from build123d import *

# Parameters (mm, degrees)
F0_W     = 40
F0_H     = 20
F1_DEPTH = 20
F3_DEPTH = 40.001


with BuildPart() as f1:
    # F0 (on Top) → F1 (new body)
    with BuildSketch(Plane.XY):
        with Locations((-41.790509, -39.392859)):
            Rectangle(F0_W, F0_H)
    extrude(amount=F1_DEPTH)

    # F2 (on face) → F3 (cut, through all)
    with BuildSketch(Plane.YZ.offset(-21.790509)):
        Polygon((-39.392859, 10), (-39.392859, 20), (-49.392859, 20), (-49.392859, 0), align=None)
    extrude(amount=-F3_DEPTH, mode=Mode.SUBTRACT)


solid = f1.part
The model under review builds one solid part; all positions refer to its coordinate system, in mm. A direction names the side the tool comes from. Coordinates: 2 decimals unless noted, no trailing zeros. Order: outer loops, then holes, each group sorted by start corner. A loop starts at its lowest first (then second) coordinate and runs counter-clockwise, first axis right, second up. Notation, with made-up numbers: (84, 65.5) -> (107, 65.5) arc R21 ccw to (107, 80.5) -> close; hole circle Ø2 at (57.25, -22). An arc over 180 degrees is marked (long way). Answer in a Markdown table with one row per item.
(1) Consider section A-A (z = 13.25). Write out the cut boundary in (x, y).
Answers:
| item | result |
|---|---|
| outline | (-61.79, -39.39) -> (-21.79, -39.39) -> (-21.79, -29.39) -> (-61.79, -29.39) -> close |
(2) Consider section C-C (y = -41.25). Write out the cut boundary in (x, z).
Answers:
| item | result |
|---|---|
| outline | (-61.79, 0) -> (-21.79, 0) -> (-21.79, 8.14) -> (-61.79, 8.14) -> close |
(3) Machinability: for faces 1 (the flat face through (-42, -39.393, 15)), 2 (the flat face through (-42, -39, 0)), which of the approach directions +Z, -Z, +X, -X, +Y, -Y give a long, thin tool a straight path to every point of the face, cutting with its end or side? Answer none if there is none.
Answers:
| item | result |
|---|---|
| face 1 | +Z, +X, -X, -Y |
| face 2 | -Z, +X, -X, +Y, -Y |
(4) Consider section B-B (x = -43.5). Write out the cut boundary in (y, z).
Answers:
| item | result |
|---|---|
| outline | (-49.39, 0) -> (-29.39, 0) -> (-29.39, 20) -> (-39.39, 20) -> (-39.39, 10) -> close |
(5) Insertion check: pin 1 (10 mm diameter, centred on x = -55.5, z = 8.5, fed in from -Y); pin 2 (5 mm diameter, centred on x = -42, z = 13, fed in from -Y). Each pin has a flat end and moves straight along its axis. Give the tip position at first contact, or say it passes through.
Answers:
| item | result |
|---|---|
| pin 1 | y = -45.89 |
| pin 2 | y = -39.39 |
(6) Wall thickness on line 1 along Y through (x, z) = (-59.5, 11.75); line 2 along Y through (x, z) = (-37, 3.5); line 3 along Z through (x, y) = (-50, -47.75): over which ranges is each line inside the solid? List them lowest first.
Answers:
| item | result |
|---|---|
| line 1 | -39.39 to -29.39 |
| line 2 | -45.89 to -29.39 |
| line 3 | 0 to 1.64 |
